Autodesk Inventor part; units mm, degrees
ref_plane "Plano de trabajo1" through (0, 0, 0) normal (0, 0, 1) x (1, 0, 0)
ref_plane "Plano de trabajo2" through (-44.5, -51.5, -48) normal (0, 0, -1) x (0, 1, 0)
ref_plane "Plano de trabajo3" through (0, 0, -45.1) normal (0, 0, 1) x (1, 0, 0)
ref_plane "Plano de trabajo1" through (0, 0, 0) normal (0, 0, 1) x (1, 0, 0)
sketch "Boceto1" plane through (0, 0, 0) normal (0, 0, 1) x (1, 0, 0)
  circle A0 centre (-34.5, -38.2272) radius 1.45
  point P0 (0, 0)
  dimension "d0" = 2.9
ref_plane "Plano de trabajo2" through (-44.5, -51.5, -48) normal (0, 0, -1) x (0, 1, 0)
extrude "Extrusión1" add sketch "Boceto1" against normal up to surface (48 mm away)
ref_plane "Plano de trabajo3" through (0, 0, -45.1) normal (0, 0, 1) x (1, 0, 0)
sketch "Boceto2" plane through (0, 0, -45.1) normal (0, 0, 1) x (1, 0, 0)
  line L0 (-32.1, -35.8272) -> (-36.9, -35.8272)
  line L1 (-36.9, -35.8272) -> (-36.9, -40.6272)
  line L2 (-36.9, -40.6272) -> (-32.1, -40.6272)
  line L3 (-32.1, -40.6272) -> (-32.1, -35.8272)
  line L4 (-32.1, -35.8272) -> (-36.9, -40.6272) construction
  line L5 (-36.9, -35.8272) -> (-32.1, -40.6272) construction
  point P0 (0, 0)
  point P1 (-34.5, -38.2272)
  dimension "d3" = 4.8
  dimension "d4" = 4.8
extrude "Extrusión2" add sketch "Boceto2" along normal blind 5
chamfer "Chaflán1" distance 0.8 angle 45 4 edges at (-36.9, -40.6272, -42.6) (-36.9, -35.8272, -42.6) (-32.1, -35.8272, -42.6) (-32.1, -40.6272, -42.6)
ref_plane "Plano de trabajo4" through (0, 0, -3.1) normal (0, 0, -1) x (-1, 0, 0)
sketch "Boceto3" plane through (0, 0, -3.1) normal (0, 0, -1) x (-1, 0, 0)
  line L0 (32.1, -39.1272) -> (36.9, -39.1272)
  line L1 (36.9, -39.1272) -> (36.9, -37.3272)
  line L2 (36.9, -37.3272) -> (32.1, -37.3272)
  line L3 (32.1, -37.3272) -> (32.1, -39.1272)
  line L4 (32.1, -39.1272) -> (36.9, -37.3272) construction
  line L5 (36.9, -39.1272) -> (32.1, -37.3272) construction
  line L6 (33.6, -40.6272) -> (35.4, -40.6272)
  line L7 (35.4, -40.6272) -> (35.4, -35.8272)
  line L8 (35.4, -35.8272) -> (33.6, -35.8272)
  line L9 (33.6, -35.8272) -> (33.6, -40.6272)
  line L10 (33.6, -40.6272) -> (35.4, -35.8272) construction
  line L11 (35.4, -40.6272) -> (33.6, -35.8272) construction
  circle A0 centre (34.5, -38.2272) radius 1.4
  point P0 (0, 0)
  point P1 (35.5724, -37.3272)
  point P2 (35.4, -37.1548)
  point P3 (33.6, -37.1548)
  point P4 (33.4276, -37.3272)
  point P5 (33.4276, -39.1272)
  point P6 (33.6, -39.2996)
  point P7 (35.4, -39.2996)
  point P8 (35.5724, -39.1272)
  dimension "d12" = 1.8
  dimension "d13" = 4.8
  dimension "d14" = 2.8
ref_plane "Plano de trabajo5" through (-39.1917, -42.9189, -7.7627) normal (0, 0, -1) x (0, 1, 0)
extrude "Extrusión3" add sketch "Boceto3" along normal up to surface (4.6627 mm away)
chamfer "Chaflán2" distance 0.2 angle 45 8 edges at (-35.4, -35.8272, -5.4314) (-36.9, -37.3272, -5.4314) (-36.9, -39.1272, -5.4314) (-35.4, -40.6272, -5.4314) (-33.6, -40.6272, -5.4314) (-33.6, -35.8272, -5.4314) (-32.1, -37.3272, -5.4314) (-32.1, -39.1272, -5.4314)
ref_plane "Plano de trabajo6" through (-34.5, -38.2272, -24) normal (0, 0, 1) x (1, 0, 0)
sketch "Boceto4" plane through (-34.5, -38.2272, -24) normal (0, 0, 1) x (1, 0, 0)
  circle A0 centre (0, 0) radius 1.55 construction
  line L0 (2.4, 3.5) -> (-2.4, 3.5)
  line L1 (-2.4, 3.5) -> (-2.4, -3.5)
  line L2 (-2.4, -3.5) -> (2.4, -3.5)
  line L3 (2.4, -3.5) -> (2.4, 3.5)
  line L4 (2.4, 3.5) -> (-2.4, -3.5) construction
  line L5 (-2.4, 3.5) -> (2.4, -3.5) construction
  point P0 (34.5, 38.2272)
  dimension "d20" = 7
  dimension "d26" = 4.8
extrude "Extrusión4" add sketch "Boceto4" along normal mid plane 10
chamfer "Chaflán3" distance 1.2 angle 45 4 edges at (-36.9, -34.7272, -24) (-36.9, -41.7272, -24) (-32.1, -34.7272, -24) (-32.1, -41.7272, -24)
sketch "Boceto5" plane through (-36.9, -40.5272, -19) normal (-1, 0, 0) x (0, 0, 1)
  line L0 (-5, 48.8726) -> (-5, -9.5454) construction
  line L1 (-5, 2.3) -> (-5, -1.2) construction
  line L2 (-10, -1.2) -> (0, -1.2) construction
  line L3 (-5, 2.3) -> (-5, 5.8) construction
  line L4 (-10, 5.8) -> (0, 5.8) construction
  point P0 (19, 40.5272)
hole "Agujero1" at (-36.9, -38.2272, -24) direction (1, 0, 0) diameter 3 end through all
properties part number "EjeEngraneGrua"
Read the model definition and answer for the solid it produces. Units are mm, in the model's axes. A direction names the side the tool comes from. Give positions to 0.01 mm unless a question says otherwise; leave off trailing zeros. Write each loop counter-clockwise with the first axis right and the second up, starting at its lowest first coordinate (ties: lowest second). Pieces come first, ordered by that corner, then holes. Notation, with made-up numbers: (18.25, 57.5) - (40.25, 57.5) arc R18 ccw to (40.25, 85.5) - close; hole circle Ø9 at (9.5, 10.25). An arc over 180 degrees is marked (long way). Answer in a Markdown table with one row per item. Add a question column.
Item 1: A tool of negligible diameter and unlimited length cuts with its end or side. For faces 1 (the face through (-35.65, -39.11, -46.53)), 2 (the face through (-35, -40.627, -43)), 3 (the face through (-36.51, -40.22, -42.64)), 4 (the face through (-36.506, -36.233, -42.565)), 5 (the face through (-35.4, -36.6, -5.4)), from which of +Z, -Z, +X, -X, +Y, -Y can it reach the whole face along a straight path? Write none if from no direction.
Item 2: Section A-A, the plane z = -24 is taken. Write down the section's boundary in (x, y).
Item 3: Flat-ended cylindrical pins translate along their axes: P1, Ø0.6, axis at x = -36.5, y = -38.5, coming from the +Z side; P2, Ø1.5, axis at x = -34.5, z = -5.5, coming from the +Y side; P3, Ø0.5, axis at x = -32.5, z = -4.5, coming from the +Y side. Find the tip coordinate at first contact, or state that the pin passes through.
Item 4: Section D-D, the plane z = -9 is taken. Write down the section's boundary in (x, y).
Item 5: Find the intervals of material crossed by L1, parallel to Z at x = -34.5, y = -36.25; L2, parallel to Z at x = -32.25, y = -39.5; L3, parallel to Y at x = -34.7, z = -24, in increasing order.
Item 6: Determine the mould class of faces 6 (the face through (-35, -40, -19)), 7 (the face through (-34, -36, -3.1)), 8 (the face through (-36, -39.127, -5)), 9 (the face through (-35.57, -37.25, -9.37)) for opening direction Z: pulls with the +Z half, pulls with the -Z half, needs draft (parallel to the pull), parting line crosses it, or undercut.
Item 7: Section C-C, the plane z = -43.5 is taken. Write down the section's boundary in (x, y), and give its area (3 significant figures).
Recorded:
| question | item | result |
|---|---|---|
| 1 | face 1 | -Z |
| 1 | face 2 | -Z, +X, -X, -Y |
| 1 | face 3 | -Z, -X, -Y |
| 1 | face 4 | -Z, -X, +Y |
| 1 | face 5 | +Z, -X, +Y |
| 2 | outline | (-36.9, -40.53) - (-35.7, -41.73) - (-33.3, -41.73) - (-32.1, -40.53) - (-32.1, -39.73) - (-36.9, -39.73) - close; (-36.9, -36.73) - (-32.1, -36.73) - (-32.1, -35.93) - (-33.3, -34.73) - (-35.7, -34.73) - (-36.9, -35.93) - close |
| 3 | P1 | stops at z = -3.1 |
| 3 | P2 | stops at y = -35.83 |
| 3 | P3 | stops at y = -37.33 |
| 4 | outline | circle Ø2.9 at (-34.5, -38.23) |
| 5 | L1 | z = -45.1 to -40.1, -29 to -19, -7.76 to -3.1 |
| 5 | L2 | z = -45.1 to -40.1, -29 to -24.79, -23.21 to -19 |
| 5 | L3 | y = -41.73 to -39.73, -36.73 to -34.73 |
| 6 | face 6 | undercut |
| 6 | face 7 | pulls with the +Z half |
| 6 | face 8 | needs draft |
| 6 | face 9 | undercut |
| 7 | outline | (-36.9, -39.83) - (-36.1, -40.63) - (-32.9, -40.63) - (-32.1, -39.83) - (-32.1, -36.63) - (-32.9, -35.83) - (-36.1, -35.83) - (-36.9, -36.63) - close |
| 7 | area | 21.8 mm2 |
